Check sheet for the modelled part. Datum: model origin and axes. Units: mm. A direction names the side the tool comes from. Coordinates: 2 decimals unless noted, no trailing zeros. Loops run counter-clockwise (first coordinate to the right, second up) from the corner with the lowest first, then second, coordinate; pieces in that order, holes last. Notation, with made-up numbers: M 66,-25.5 L 90,-25.5 A21 cw 90,7.5 Z; hole C 74.25,47.25 d1. An arc over 180 degrees is marked long. Return JSON: item names as keys, results as strings.
from build123d import *

# Parameters (mm, degrees)
SKETCH_2_W          = 24
SKETCH_2_H          = 12.5
SKETCH_2_W_2        = 32
FILLET_2_R          = 0.02
CUT_EXTRUDE_1_DEPTH = 20
CUT_EXTRUDE_2_DEPTH = 20
EXTRUDE_2_DEPTH     = 12.5
CHAMFER_3_SIZE      = 2


with BuildPart() as part:
    # 草图2 → 旋转1 (revolve)
    with BuildSketch(Plane(origin=(0, 0, 0), x_dir=(1, 0, 0), z_dir=(0, 1, 0)), mode=Mode.PRIVATE) as revolve_1_sk:
        with Locations((-68, 6.25)):
            Rectangle(SKETCH_2_W, SKETCH_2_H)
        Polygon((-56, 0), (-50, 0), (-50, 17.5), (-50, 20), (-56, 20), (-56, 12.5), align=None)
        Polygon((-50, 0), (0, 0), (0, 12.5), (0, 17.5), (-50, 17.5), align=None)
        with Locations((16, 6.25)):
            Rectangle(SKETCH_2_W_2, SKETCH_2_H)
        Polygon((52, 0), (52, 7.5), (52, 11.5), (32, 11.5), (32, 0), align=None)
        with BuildLine():
            ThreePointArc((56, 6.5), (56.707106781, 6.792893219), (57, 7.5))
            Line((57, 7.5), (57, 0))
            Line((57, 0), (52, 0))
            Line((52, 0), (52, 7.5))
            ThreePointArc((52, 7.5), (52.292893219, 6.792893219), (53, 6.5))
            Line((53, 6.5), (56, 6.5))
        make_face()
        Polygon((57, 8), (57, 7.5), (57, 0), (80, 0), (80, 8), align=None)
    revolve(revolve_1_sk.sketch.rotate(Axis((-92.921580587, 0, 0), (1, 0, 0)), 180), axis=Axis((-92.921580587, 0, 0), (1, 0, 0)))

    # 倒角2: read off the stored shape, not the designer's step
    # 倒角2 outline → 倒角2 (revolve, cut)
    with BuildSketch(Plane.YX):
        Polygon((7, 56.866025404), (7.5, 56.866025404), (7.5, 57), (8, 57), (8, 58.598076211), align=None)
        Polygon((17.5, 0), (15.5, 0), (17.5, -2), align=None)
    revolve(axis=Axis((0, 0, 0), (1, 0, 0)), mode=Mode.SUBTRACT)

    # 圆角2
    fillet_2_edges = [part.edges().sort_by_distance(p)[0] for p in [
        (-50, 0, -20),
    ]]
    fillet(fillet_2_edges, radius=FILLET_2_R)

    # 草图3 → 切除-拉伸1 (cut)
    with BuildSketch(Plane(origin=(52, 0, 0), x_dir=(0, 0, -1), z_dir=(1, 0, 0))):
        Polygon((13.451018428, -3.326790062), (11.426075214, -1.301846848), (1.301846848, -11.426075214), (3.326790062, -13.451018428), align=None)
        Polygon((1.301846848, 11.426075214), (11.426075214, 1.301846848), (13.451018428, 3.326790062), (3.326790062, 13.451018428), align=None)
        Polygon((-13.451018428, 3.326790062), (-11.426075214, 1.301846848), (-1.301846848, 11.426075214), (-3.326790062, 13.451018428), align=None)
        Polygon((-1.301846848, -11.426075214), (-3.326790062, -13.451018428), (-13.451018428, -3.326790062), (-11.426075214, -1.301846848), align=None)
    extrude(amount=-CUT_EXTRUDE_1_DEPTH, mode=Mode.SUBTRACT)

    # 草图5 → 切除-拉伸2 (cut)
    with BuildSketch(Plane.XY):
        with BuildLine():
            Line((-33.02, 5), (-17.02, 5))
            ThreePointArc((-17.02, 5), (-12.02, 0), (-17.02, -5))
            Line((-17.02, -5), (-33.02, -5))
            ThreePointArc((-33.02, -5), (-38.02, 0), (-33.02, 5))
        make_face()
    extrude(amount=-CUT_EXTRUDE_2_DEPTH, mode=Mode.SUBTRACT)

    # 草图4 → 凸台-拉伸2 (add)
    with BuildSketch(Plane.XY):
        with BuildLine():
            Line((-33.02, 5), (-17.02, 5))
            ThreePointArc((-17.02, 5), (-12.02, 0), (-17.02, -5))
            Line((-17.02, -5), (-33.02, -5))
            ThreePointArc((-33.02, -5), (-38.02, 0), (-33.02, 5))
        make_face()
    extrude(amount=-EXTRUDE_2_DEPTH)

    # 倒角3
    chamfer_3_edges = [part.edges().sort_by_distance(p)[0] for p in [
        (-80, 0, -12.5),
    ]]
    chamfer(chamfer_3_edges, length=CHAMFER_3_SIZE)


solid = part.part
1) Go/stop test with flat-tipped pins: pin 1 Ø6 at (y, z) = (-15.5, -9.5) entering from -X; pin 2 Ø8 at (x, z) = (-32, -11) entering from -Y; pin 3 Ø10 at (y, z) = (15.5, 11) entering from +X. Record where each tip stops, or that it passes through.
Answers:
{"pin 1": "x = -56", "pin 2": "y = -16.04", "pin 3": "x = 0"}
2) Section check A-A on x = 50.5. Record the cut outline in (y, z), then the cut area to 3 significant figures.
Answers:
{"outline": "M -11.43,-1.3 L -1.3,-11.43 A11.5 ccw 1.3,-11.43 L 11.43,-1.3 A11.5 ccw 11.43,1.3 L 1.3,11.43 A11.5 ccw -1.3,11.43 L -11.43,1.3 A11.5 ccw Z", "area": "318 mm²"}
3) Section check C-C on x = 8. Record the cut outline in (y, z), then the cut area to 3 significant figures.
Answers:
{"outline": "C 0,0 d25", "area": "491 mm²"}
4) Draft check along Y on faces 4 (the face through (-0.125, -3.387, -15.254)), 5 (the face through (-38.02, -0.11, -14.97)), 6 (the face through (80, 0, 0)). Enter one of: +Y half, -Y half, draft (parallel to the pull), parting line (faces both ways), or undercut.
Answers:
{"face 4": "parting line", "face 5": "undercut", "face 6": "draft"}
5) Scan lines: line 1 along X through (y, z) = (1, 18.5); line 2 along X through (y, z) = (-7, 12.5); line 3 along Y through (x, z) = (-21, -13.5). Record each from-to range of solid material in increasing order. Write a range as [from, to].
Answers:
{"line 1": "[-56, -50]", "line 2": "[-56, 0]", "line 3": "[-11.14, -5], [5, 11.14]"}
6) Section check B-B on x = 66.5. Record the cut outline in (y, z).
Answers:
{"outline": "C 0,0 d16"}
7) Set-up check for faces 1 (the face through (42.14, 6.435, -6.293)), 2 (the face through (52, 1, -8)), 3 (the face through (-26.34, -5.26, 16.69)): record each of +Z, -Z, +X, -X, +Y, -Y from which the full face is reachable in a straight line by a thin tool's end or side.
Answers:
{"face 1": "-Z, +X, +Y", "face 2": "none", "face 3": "+X"}
